Read the model definition and answer for the solid it produces. Units are mm, in the model's axes. Face numbers are marked on the shaded views. A direction names the side the tool comes from. Coordinates: 2 decimals unless noted, no trailing zeros. Loops run counter-clockwise (first coordinate to the right, second up) from the corner with the lowest first, then second, coordinate; pieces in that order, holes last. Notation, with made-up numbers: M 67.25,79.5 L 91.25,79.5 A14 ccw 91.25,105.5 Z; hole C 37,-39 d6. An arc over 180 degrees is marked long. Use one line per item in the form item = value. Start each with the question number.
1. A tool of negligible diameter and unlimited length cuts with its end or side. For the marked faces 1 and 2, from which of +Z, -Z, +X, -X, +Y, -Y can it reach the whole face along a straight path? Write none if from no direction.
2. The part is cut by section C-C (y = -5.75). Give the vertices of the cut face in (x, z).
3. The part is cut by section A-A (z = 58). Give the vertices of the cut face in (x, y).
4. The part is cut by section B-B (x = 5.5). Give the vertices of the cut face in (y, z), plus the area to 3 significant figures.
5. Flat-ended cylindrical pins translate along their axes: pin 1 (5 mm diameter, centred on y = 4.5, z = 9.5, fed in from -X); pin 2 (3 mm diameter, centred on x = -1, y = -4, fed in from +Z); pin 3 (2 mm diameter, centred on x = 0, z = 58.5, fed in from +Y). Find the tip coordinate at first contact, or state that the pin passes through.
6. The part is cut by section D-D (z = 31). Give the vertices of the cut face in (x, y), plus the area to 3 significant figures.
7. Find the intervals of material crossed by probe 1 along Z at (x, y) = (-4, -6); probe 2 along Y at (x, z) = (0.25, 36); probe 3 along Y at (x, z) = (4, 17.5), in increasing order. Write a range as [from, to].
from build123d import *

# Parameters (mm, degrees)
SKETCH2_R           = 7.25
BOSS_EXTRUDE1_DEPTH = 41
BOSS_EXTRUDE2_DEPTH = 6
SKETCH4_R           = 2.34
BOSS_EXTRUDE3_DEPTH = 18.67
FILLET1_R           = 1
SKETCH5_R           = 1.5
BOSS_EXTRUDE4_DEPTH = 4.42


with BuildPart() as part:
    # Sketch2 → Boss-Extrude1 (new body)
    with BuildSketch(Plane.XY):
        Circle(SKETCH2_R)
    extrude(amount=BOSS_EXTRUDE1_DEPTH)

    # Sketch3 → Boss-Extrude2 (add)
    with BuildSketch(Plane.XY.offset(41)):
        Polygon((3.031985372, -1.675429707), (2.966957375, 1.788061503), (-0.065027998, 3.46349121), (-3.031985372, 1.675429707), (-2.966957375, -1.788061503), (0.065027998, -3.46349121), align=None)
    extrude(amount=BOSS_EXTRUDE2_DEPTH)

    # Sketch4 → Boss-Extrude3 (add)
    with BuildSketch(Plane.XY.offset(47)):
        Circle(SKETCH4_R)
    extrude(amount=BOSS_EXTRUDE3_DEPTH)

    # Fillet1
    fillet1_edges = [part.edges().sort_by_distance(p)[0] for p in [
        (-2.34, 0, 47),
    ]]
    fillet(fillet1_edges, radius=FILLET1_R)

    # Sketch5 → Boss-Extrude4 (add)
    with BuildSketch(Plane.XY.offset(65.67)):
        Circle(SKETCH5_R)
    extrude(amount=BOSS_EXTRUDE4_DEPTH)


solid = part.part
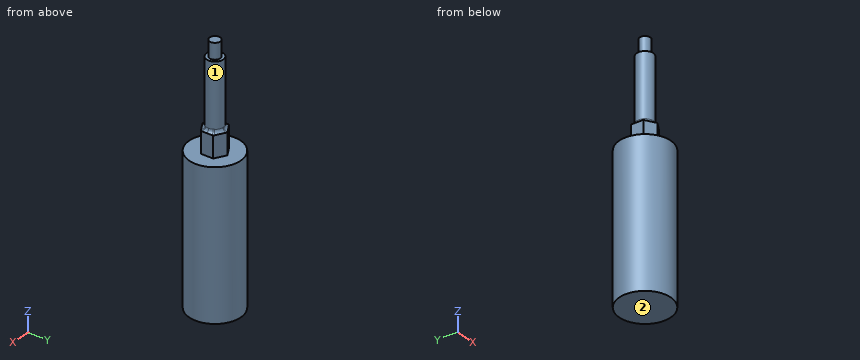
Computed values:
q1.face_1 = +Z
q1.face_2 = -Z, +X, -X, +Y, -Y
q2.outline = M -4.42,0 L 4.42,0 L 4.42,41 L -4.42,41 Z
q3.outline = C 0,0 d4.68
q4.outline = M -4.72,0 L 4.72,0 L 4.72,41 L -4.72,41 Z
q4.area = 387 mm²
q5.pin_1 = -6.97
q5.pin_2 = 47.28
q5.pin_3 = 2.34
q6.outline = C 0,0 d14.5
q6.area = 165 mm²
q7.probe_1 = [0, 41]
q7.probe_2 = [-7.25, 7.25]
q7.probe_3 = [-6.05, 6.05]
